Work out the finished part from the listing and answer in its coordinate system (mm). Face numbers are marked on the shaded views. A direction names the side the tool comes from. Round coordinates to 2 decimals unless told otherwise and drop trailing zeros. Order: outer loops, then holes, each group sorted by start corner. A loop starts at its lowest first (then second) coordinate and runs counter-clockwise, first axis right, second up. Notation, with made-up numbers: (20, 89) - (49, 89) arc R25 ccw to (49, 118) - close; hole circle Ø1 at (25, 1.25). An arc over 180 degrees is marked (long way). Answer in a Markdown table with one row per item.
from build123d import *

# Parameters (mm, degrees)
SKETCH_6_W      = 80
SKETCH_6_H      = 40
SKETCH_6_W_2    = 76
SKETCH_6_H_2    = 36
SKETCH_14_W     = 40
SKETCH_14_H     = 80
EXTRUDE_1_DEPTH = 194
SKETCH_15_W     = 80
SKETCH_15_H     = 40
EXTRUDE_2_DEPTH = 595


with BuildPart() as part:
    # По траектории13: sweep along a curve in space
    with BuildLine() as sweep_13_path:
        Line((0, 0, 0), (1000, 0, 0))
        Line((1000, 0, 0), (1000, -150, 0))
        Line((1000, -150, 0), (566.987298108, -400, 0))
        Line((566.987298108, -400, 0), (263.878406783, -225, 0))
        Line((263.878406783, -225, 0), (0, -147.584326952, 0))
        Line((0, -147.584326952, 0), (0, 0, 0))
    # Эскиз6 → По траектории13 (sweep)
    with BuildSketch(Plane(origin=(0, 0, 0), x_dir=(0, 0, -1), z_dir=(1, 0, 0))):
        with Locations((-0.551773823, -1.216505436)):
            Rectangle(SKETCH_6_W, SKETCH_6_H)
        with Locations((-0.551773823, -1.216505436)):
            Rectangle(SKETCH_6_W_2, SKETCH_6_H_2, mode=Mode.SUBTRACT)
    sweep(path=sweep_13_path.line, transition=Transition.RIGHT)

    # Эскиз14 → Бобышка-Вытянуть1 (add)
    with BuildSketch(Plane(origin=(-33.89376203, -115.529989888, 0), x_dir=(0.9595578428480989, -0.2815115383580276, 0), z_dir=(0.2815115383580276, 0.9595578428480989, 0))):
        with Locations((299.085913187, -0.551773823)):
            Rectangle(SKETCH_14_W, SKETCH_14_H)
    extrude(amount=EXTRUDE_1_DEPTH)

    # Эскиз15 → Бобышка-Вытянуть2 (add)
    with BuildSketch(Plane(origin=(306.181390541, -89.82636629, 0), x_dir=(0, 0, -1), z_dir=(0.9595578428480989, -0.28151153835802767, 0))):
        with Locations((-0.551773823, 51.50143726)):
            Rectangle(SKETCH_15_W, SKETCH_15_H)
    extrude(amount=EXTRUDE_2_DEPTH)


solid = part.part
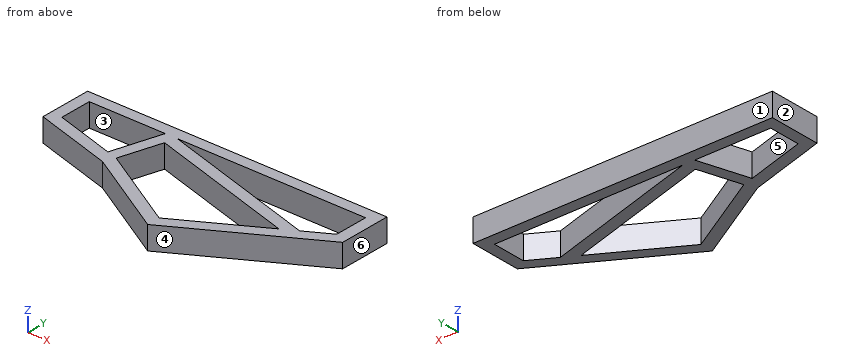
1) Each of these flat-tipped pins is pushed along its axis until it touches: pin 1 (5 mm diameter, centred on y = -321.5, z = -7, fed in from -X); pin 2 (3 mm diameter, centred on y = -293, z = -19, fed in from +X); pin 3 (5 mm diameter, centred on x = 864.5, z = -8.5, fed in from -Y). Where does it stop, or does it pass through?
Filled in:
| item | result |
|---|---|
| pin 1 | stops at x = 389.12 |
| pin 2 | stops at x = 792.48 |
| pin 3 | stops at y = -251.36 |
2) Find section D-D, the plane z = -5. Give the number of separate pieces and of enclosed holes in the cut face, then the cut area to 3 significant figures.
Filled in:
| item | result |
|---|---|
| separate pieces | 2 |
| enclosed holes | 4 |
| area | 41,000 mm^2 |
3) Find section C-C, the plane x = 640. Give the vertices of the cut face in (y, z).
Filled in:
| item | result |
|---|---|
| outline | (-379.54, -39.45) - (-333.35, -39.45) - (-333.35, 40.55) - (-379.54, 40.55) - close; (-154.93, -39.45) - (-113.25, -39.45) - (-113.25, 40.55) - (-154.93, 40.55) - close; (-21.22, -39.45) - (18.78, -39.45) - (18.78, 40.55) - (-21.22, 40.55) - close; hole (-377.23, -37.45) - (-335.66, -37.45) - (-335.66, 38.55) - (-377.23, 38.55) - close; hole (-19.22, -37.45) - (16.78, -37.45) - (16.78, 38.55) - (-19.22, 38.55) - close |
4) The mould has two halves that part along Y. Classify the marked faces 1, 2, 3 and 4: released by +Y, released by -Y, zero draft, split by the parting line, or undercut.
Filled in:
| item | result |
|---|---|
| face 1 | released by +Y |
| face 2 | zero draft |
| face 3 | undercut |
| face 4 | released by -Y |
5) Find the intervals of material crossed by probe 1 along X at (y, z) = (-20, 35.5); probe 2 along Y at (x, z) = (105, 20); probe 3 along Y at (x, z) = (549.5, -15) (1 decimal), in increasing order. Write a range as from..to.
Filled in:
| item | result |
|---|---|
| probe 1 | x = -18.78..-16.78, 19.22..980.78, 1016.78..1018.78 |
| probe 2 | y = -197.96..-195.88, -158.36..-156.28, -21.22..-19.22, 16.78..18.78 |
| probe 3 | y = -411.6..-409.3, -367.7..-365.4, -128.4..-86.7, -21.2..-19.2, 16.8..18.8 |
6) Find section A-A, the plane x = 44.5. Give the vertices of the cut face in (y, z).
Filled in:
| item | result |
|---|---|
| outline | (-180.21, -39.45) - (-138.53, -39.45) - (-138.53, 40.55) - (-180.21, 40.55) - close; (-21.22, -39.45) - (18.78, -39.45) - (18.78, 40.55) - (-21.22, 40.55) - close; hole (-178.13, -37.45) - (-140.61, -37.45) - (-140.61, 38.55) - (-178.13, 38.55) - close; hole (-19.22, -37.45) - (16.78, -37.45) - (16.78, 38.55) - (-19.22, 38.55) - close |
7) Which of the six approach directions +Z, -Z, +X, -X, +Y, -Y give full straight-line access (tool end or side, diameter ignored) to the marked faces 5 and 6?
Filled in:
| item | result |
|---|---|
| face 5 | +Z, -Z |
| face 6 | +Z, -Z, +X, +Y, -Y |
8) Find section B-B, the plane y = -265. Give the vertices of the cut face in (x, z), then the cut area to 3 significant figures.
Filled in:
| item | result |
|---|---|
| outline | (295.59, -39.45) - (375.59, -39.45) - (375.59, 40.55) - (295.59, 40.55) - close; (758.38, -39.45) - (838.38, -39.45) - (838.38, 40.55) - (758.38, 40.55) - close; hole (299.59, -37.45) - (371.59, -37.45) - (371.59, 38.55) - (299.59, 38.55) - close; hole (762.38, -37.45) - (834.38, -37.45) - (834.38, 38.55) - (762.38, 38.55) - close |
| area | 1,860 mm^2 |
